Build history of the part. All positions in model axes, mm. Round coordinates to 2 decimals unless told otherwise and drop trailing zeros. Write each loop counter-clockwise with the first axis right and the second up, starting at its lowest first coordinate (ties: lowest second). Pieces come first, ordered by that corner, then holes. Notation, with made-up numbers: (83.25, -39) -> (116.25, -39) arc R20 ccw to (116.25, -11) -> close; hole circle Ø6 at (36.5, 47). An arc over 180 degrees is marked (long way). Answer as CSV lines item,"result".
from build123d import *

# Parameters (mm, degrees)
SKETCH1_R           = 1.5
BOSS_EXTRUDE1_DEPTH = 2.25
FILLET1_R           = 0.1


with BuildPart() as part:
    # Sketch1 → Boss-Extrude1 (new body)
    with BuildSketch(Plane(origin=(0, 0, 0), x_dir=(1, 0, 0), z_dir=(0, 1, 0))):
        Polygon((2.739003368, -1.606609438), (2.760866271, 1.568741778), (0.021862903, 3.175351216), (-2.739003368, 1.606609438), (-2.760866271, -1.568741778), (-0.021862903, -3.175351216), align=None)
        with Locations(Location((0, 0, 0), (0, 0, 270))):
            Circle(SKETCH1_R, mode=Mode.SUBTRACT)
    extrude(amount=BOSS_EXTRUDE1_DEPTH)

    # Fillet1
    fillet1_edges = [part.edges().sort_by_distance(p)[0] for p in [
        (1.391364587, 2.25, -2.372046497),
        (-1.358570232, 2.25, -2.390980327),
        (-2.749934819, 2.25, -0.01893383),
        (0, 0, -1.5),
        (0, 2.25, -1.5),
        (-1.391364587, 2.25, 2.372046497),
        (1.358570232, 2.25, 2.390980327),
        (-1.391364587, 0, 2.372046497),
        (-2.749934819, 0, -0.01893383),
        (-1.358570232, 0, -2.390980327),
        (2.749934819, 2.25, 0.01893383),
        (1.391364587, 0, -2.372046497),
        (2.749934819, 0, 0.01893383),
        (1.358570232, 0, 2.390980327),
    ]]
    fillet(fillet1_edges, radius=FILLET1_R)


solid = part.part
1. Mould opens along X. For faces 1 (the flat face through (1.41, 1.11, -2.36)), 2 (the flat face through (-1.34, 1.11, -2.4)), 3 (the cylindrical face through (0.45, 1.11, 1.43)) say: +X half, -X half, draft (parallel to the pull), parting line (faces both ways), or undercut.
Results found:
face 1,"+X half"
face 2,"-X half"
face 3,"undercut"
2. Cut at A-A, the plane y = 0.6. Write the cut outline in (x, z), then the cut area to 3 significant figures.
Results found:
outline,"(-2.76, 1.57) -> (-2.74, -1.61) -> (0.02, -3.18) -> (2.76, -1.57) -> (2.74, 1.61) -> (-0.02, 3.18) -> close; hole circle Ø3 at (0, 0)"
area,"19.1 mm2"
3. Probe line 1 along X through (y, z) = (2, -2.25); line 2 along X through (y, z) = (1.3, 0); line 3 along X through (y, z) = (0.5, -0.5). List the from-to ranges inside material, lowest first.
Results found:
line 1,"x = -1.61 to 1.6"
line 2,"x = -2.75 to -1.5, 1.5 to 2.75"
line 3,"x = -2.75 to -1.41, 1.41 to 2.75"
